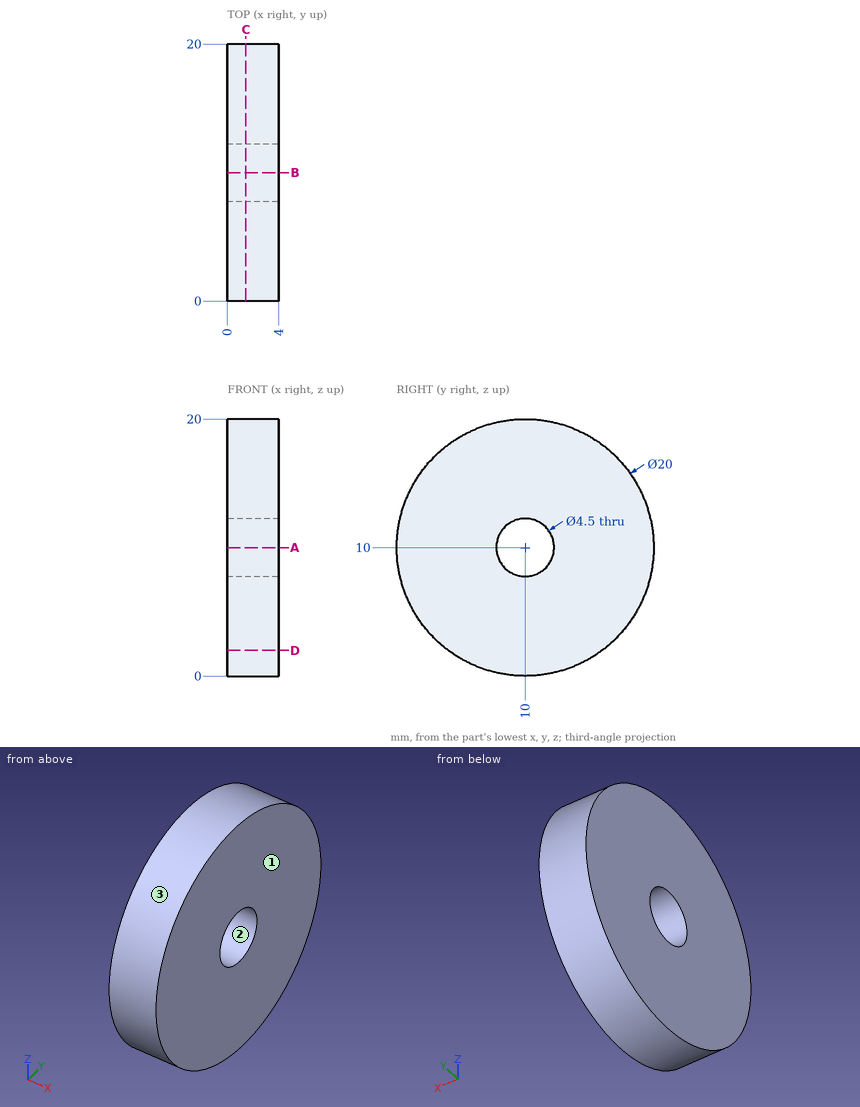
Design review of the part shown in the three views and the two pictorial views. Dimensions are in mm from the part's minimum x, y and z. Give positions to 0.01 mm unless a question says otherwise; leave off trailing zeros. Write each loop counter-clockwise with the first axis right and the second up, starting at its lowest first coordinate (ties: lowest second). Pieces come first, ordered by that corner, then holes. Notation, with made-up numbers: (88.25, 57.25) - (107.25, 57.25) arc R14 cw to (107.25, 70.25) - close; hole circle Ø5 at (-26, -34.5). An arc over 180 degrees is marked (long way). Return JSON: item names as keys, results as strings. Group by question number.
(1) We need section D-D, the plane z = 2. Give the boundary of the cut face in (x, y), then the cut area to 3 significant figures.
(2) Insertion check: pin 1 (5 mm diameter, centred on y = 10, z = 10, fed in from -X). The pin has a flat end and moves straight along its axis. Give the tip position at first contact, or say it passes through.
(3) We need section C-C, the plane x = 1.45. Give the boundary of the cut face in (y, z), then the cut area to 3 significant figures.
(4) Mouldability with a two-part tool opening along Y and no side actions: class the marked faces 1, 2 and 3 as +Y half, -Y half, draft (parallel to the pull), parting line (faces both ways), or undercut.
(5) We need section A-A, the plane z = 10. Give the boundary of the cut face in (x, y), then the cut area to 3 significant figures.
(6) To check wall thickness, follow probe 1 along Z at (x, y) = (2.1, 10); probe 2 along Y at (x, z) = (3.7, 11.75). State the ranges of each line that lie inside material, in increasing order.
Reported:
{
 "1": {"outline": "(0, 4) - (4, 4) - (4, 16) - (0, 16) - close", "area": "48.0 mm2"},
 "2": {"pin 1": "stops at x = 0"},
 "3": {"outline": "circle Ø20 at (10, 10); hole circle Ø4.5 at (10, 10)", "area": "298 mm2"},
 "4": {"face 1": "draft", "face 2": "undercut", "face 3": "parting line"},
 "5": {"outline": "(0, 0) - (4, 0) - (4, 7.75) - (0, 7.75) - close; (0, 12.25) - (4, 12.25) - (4, 20) - (0, 20) - close", "area": "62.0 mm2"},
 "6": {"probe 1": "z = 0 to 7.75, 12.25 to 20", "probe 2": "y = 0.15 to 8.59, 11.41 to 19.85"}
}
